from build123d import *

# Parameters (mm, degrees)
F0_R     = 63.5
F1_DEPTH = 25.4
F2_W     = 25.4
F2_H     = 25.4
F3_DEPTH = 50.801


with BuildPart() as f1:
    # F0 (on Front) → F1 (new body, symmetric)
    with BuildSketch(Plane.XZ):
        Circle(F0_R)
    extrude(amount=F1_DEPTH, both=True)

    # F2 (on face) → F3 (cut, through all)
    with BuildSketch(Plane.XZ.offset(25.4)):
        Rectangle(F2_W, F2_H)
    extrude(amount=-F3_DEPTH, mode=Mode.SUBTRACT)


solid = f1.part
The model under review builds one solid part; all positions refer to its coordinate system, in mm. A direction names the side the tool comes from. Coordinates: 2 decimals unless noted, no trailing zeros. Loops run counter-clockwise (first coordinate to the right, second up) from the corner with the lowest first, then second, coordinate; pieces in that order, holes last. Notation, with made-up numbers: M -32,-8.5 L 24,-8.5 A11 cw 24,3.5 Z; hole C -23.5,41.5 d7. An arc over 180 degrees is marked long. Put each result on its own line as item: value. Start each with the question number.
Q1. Add section A-A (x = 0). Write out the cut boundary in (y, z).
Q2. The part is to be moulded in two halves that separate along Z. For faces 1 (the flat face through (13, -25.4, 1)), 2 (the cylindrical face through (-13.77, -0.36, -61.99)), 3 (the flat face through (-12.7, 0, 0)), say which applies: +Z half, -Z half, draft (parallel to the pull), parting line (faces both ways), or undercut.
Q3. Add section B-B (z = 0). Write out the cut boundary in (x, y).
Q4. For faces 4 (the flat face through (12.7, 0, 0)), 5 (the flat face through (13, 25.4, 1)), list the 3-axis set-ups (+Z, -Z, +X, -X, +Y, -Y) from which the entire face can be reached by the end or side of a thin tool; tool diameter is ignored.
Q5. Add section D-D (z = 40.5). Write out the cut boundary in (x, y), and give its area (3 significant figures).
Q6. Clearance check with flat-ended pins moving along their axes: pin 1 (5 mm diameter, centred on y = 15, z = -40.5, fed in from -X); pin 2 (1 mm diameter, centred on x = -50, y = -2, fed in from -Z); pin 3 (20.5 mm diameter, centred on x = 4.5, y = 4, fed in from +Z). State where each tip first meets the part, or that it passes through.
Q7. Add section C-C (y = 8). Write out the cut boundary in (x, z).
Q8. Wall thickness on line 1 (X direction, y = -13, z = 6.5); line 2 (X direction, y = -6, z = -10); line 3 (Z direction, x = -5, y = -6): over which ranges is each line inside the solid? List them lowest first.
Answers:
1. outline: M -25.4,-63.5 L 25.4,-63.5 L 25.4,-12.7 L -25.4,-12.7 Z; M -25.4,12.7 L 25.4,12.7 L 25.4,63.5 L -25.4,63.5 Z
2. face 1: draft
2. face 2: parting line
2. face 3: undercut
3. outline: M -63.5,-25.4 L -12.7,-25.4 L -12.7,25.4 L -63.5,25.4 Z; M 12.7,-25.4 L 63.5,-25.4 L 63.5,25.4 L 12.7,25.4 Z
4. face 4: +Y, -Y
4. face 5: +Z, -Z, +X, -X, +Y
5. outline: M -48.91,-25.4 L 48.91,-25.4 L 48.91,25.4 L -48.91,25.4 Z
5. area: 4,970 mm^2
6. pin 1: stops at x = -50.87
6. pin 2: stops at z = -39.77
6. pin 3: stops at z = 63.5
7. outline: C 0,0 d127; hole M -12.7,-12.7 L 12.7,-12.7 L 12.7,12.7 L -12.7,12.7 Z
8. line 1: x = -63.17 to -12.7, 12.7 to 63.17
8. line 2: x = -62.71 to -12.7, 12.7 to 62.71
8. line 3: z = -63.3 to -12.7, 12.7 to 63.3
